Design review of the part built by this model. Coordinates are the model's own, in mm. Face numbers are marked on the shaded views. A direction names the side the tool comes from. Coordinates: 2 decimals unless noted, no trailing zeros. Order: outer loops, then holes, each group sorted by start corner. A loop starts at its lowest first (then second) coordinate and runs counter-clockwise, first axis right, second up. Notation, with made-up numbers: (-39.75, 12) -> (13.25, 12) arc R22 cw to (13.25, 37) -> close; hole circle Ø11 at (48, 61). An arc over 180 degrees is marked (long way). Use a Markdown table: item, result. Add a question column.
Q1. Wall thickness on probe 1 along Y at (x, z) = (-29, -15); probe 2 along Y at (x, z) = (5.5, -2.5); probe 3 along X at (y, z) = (20, -0.5): over which ranges is each line inside the solid? List them lowest first.
Q2. Add section D-D (y = 48.5). State the section outline as (x, z) points.
Q3. Add section C-C (y = -14). State the section outline as (x, z) points, then the cut area to 3 significant figures.
Q4. The part is to be moulded in two halves that separate along X. For the marked faces 1, 2, 3 and 4, say which applies: pulls with the +X half, pulls with the -X half, needs draft (parallel to the pull), parting line crosses it, or undercut.
Q5. Insertion check: pin 1 (6 mm diameter, centred on x = -4.5, y = 3.5, fed in from +Z); pin 2 (8.5 mm diameter, centred on x = -21, y = -3, fed in from +Z); pin 3 (2 mm diameter, centred on x = -37, z = -35, fed in from +Y) (3 decimals); pin 4 (1.5 mm diameter, centred on x = -10.5, y = -11.5, fed in from +Z). Each pin has a flat end and moves straight along its axis. Give the tip position at first contact, or say it passes through.
Q6. Machinability: for the marked faces 5, 6, 7, 8 and 9, which of the approach directions +Z, -Z, +X, -X, +Y, -Y give a long, thin tool a straight path to every point of the face, cutting with its end or side? Answer none if there is none.
Autodesk Inventor part; units mm, degrees
ref_plane "YZ Plane" through (0, 0, 0) normal (1, 0, 0) x (0, 1, 0)
ref_plane "XZ Plane" through (0, 0, 0) normal (0, 1, 0) x (-1, 0, 0)
ref_plane "XY Plane" through (0, 0, 0) normal (0, 0, 1) x (1, 0, 0)
sketch "Sketch1" plane through (0, 0, 0) normal (0, 0, 1) x (1, 0, 0)
  line L0 (0, 0) -> (0, 60.96)
  line L1 (0, 60.96) -> (25.4, 60.96)
  arc A0 (28.575, 57.785) -> (25.4, 60.96) centre (25.4, 57.785) ccw
  line L2 (28.575, 57.785) -> (28.575, 0)
  line L3 (28.575, 0) -> (0, 0)
  dimension "d0" = 3.175
  dimension "d1" = 60.96
  dimension "d3" = 28.575
revolve "Can" add sketch "Sketch1" angle 360 about axis through (0, 0, 0) along (0, 1, 0)
sketch "Sketch2" plane through (0, 0, 0) normal (0, -1, 0) x (1, 0, 0)
  circle A0 centre (0, 0) radius 28.575
  circle A1 centre (0, 0) radius 34.036
  line L0 (-26.3398, 32.6898) -> (26.3398, 32.6898)
  line L1 (32.6898, 26.3398) -> (32.6898, -26.3398)
  line L2 (26.3398, -32.6898) -> (-26.3398, -32.6898)
  line L3 (-32.6898, -26.3398) -> (-32.6898, 26.3398)
  arc A2 (32.6898, 26.3398) -> (26.3398, 32.6898) centre (26.3398, 26.3398) ccw
  arc A3 (-26.3398, 32.6898) -> (-32.6898, 26.3398) centre (-26.3398, 26.3398) ccw
  arc A4 (-32.6898, -26.3398) -> (-26.3398, -32.6898) centre (-26.3398, -26.3398) ccw
  arc A5 (26.3398, -32.6898) -> (32.6898, -26.3398) centre (26.3398, -26.3398) ccw
  point P0 (-32.6898, 32.6898)
  point P1 (32.6898, 32.6898)
  point P2 (0, 32.6898)
  point P3 (-32.6898, 0)
  dimension "d5" = 65.3796
  dimension "d6" = 68.072
  dimension "d7" = 6.35
extrude "Plate" add sketch "Sketch2" along normal blind 10.3632 contours A0 | A1 L1 | L1 A1 L2 L3 L0 | A1 L0 A2 L1 | L1 A5 L2 A1 | L0 A1 | A1 L2 | A1 L3 A3 L0 | L2 A4 L3 A1 | L3 A1
sketch "Sketch3" plane through (0, -10.3632, 0) normal (0, -1, 0) x (1, 0, 0)
  arc A0 (-9.4777, -32.6898) -> (9.4777, -32.6898) centre (0, 0) ccw
  circle A1 centre (-16.1798, 0) radius 2.413
  circle A2 centre (16.1798, 0) radius 2.413
  dimension "d10" = 4.826
  dimension "d11" = 32.3596
  dimension "d12" = 16.1798
extrude "Coil Studs" add sketch "Sketch3" along normal blind 9.525
thread "Coil Stud 1"
thread "Coil Stud 2"
sketch "Sketch4" plane through (0, -10.3632, 0) normal (0, -1, 0) x (1, 0, 0)
  arc A0 (-9.4777, -32.6898) -> (9.4777, -32.6898) centre (0, 0) ccw
  circle A1 centre (0, 14.6812) radius 3.9688
  circle A2 centre (0, -14.6812) radius 3.9688
  dimension "d19" = 29.3624
  dimension "d20" = 14.6812
  dimension "d21" = 7.9375
extrude "Power Studs" add sketch "Sketch4" along normal blind 15.0876
thread "Power Stud 1"
thread "Power Stud 2"
ref_plane "Work Plane1" through (0, 15.24, 0) normal (0, 1, 0) x (1, 0, 0)
sketch "Sketch5" plane through (0, 15.24, 0) normal (0, 1, 0) x (1, 0, 0)
  line L0 (-37.592, 12.4714) -> (-19.05, 12.4714)
  line L1 (-19.05, 12.4714) -> (-19.05, -12.4714)
  line L2 (-19.05, -12.4714) -> (-37.592, -12.4714)
  line L3 (-37.592, -12.4714) -> (-37.592, 12.4714)
  point P0 (0, 0)
  point P1 (-19.05, 0)
  dimension "d29" = 37.592
  dimension "d30" = 24.9428
  dimension "d31" = 19.05
extrude "Extrusion4" add sketch "Sketch5" along normal blind 34.925
sketch "Sketch6" plane through (0, 50.165, 0) normal (0, 1, 0) x (1, 0, 0)
  arc A0 (-25.7098, 12.4714) -> (-25.7098, -12.4714) centre (0, 0) ccw
  line L0 (-37.592, 12.4714) -> (-25.7098, 12.4714)
  line L1 (-25.7098, -12.4714) -> (-37.592, -12.4714)
  line L2 (-37.592, 12.4714) -> (-35.7632, 12.4714)
  line L3 (-35.7632, 13.97) -> (-35.7632, 39.6951)
  line L4 (-35.7632, 39.6951) -> (-37.592, 39.6951)
  line L5 (-37.592, 39.6951) -> (-37.592, 12.4714)
  circle A1 centre (0, 0) radius 28.575
  arc A2 (-26.8755, -13.97) -> (-26.8755, 13.97) centre (0, 0) ccw
  line L6 (-35.7632, 13.97) -> (-26.8755, 13.97)
  line L7 (-37.592, -12.4714) -> (-35.7632, -12.4714)
  line L8 (-35.7632, -13.97) -> (-35.7632, -39.6951)
  line L9 (-35.7632, -39.6951) -> (-37.592, -39.6951)
  line L10 (-37.592, -39.6951) -> (-37.592, -12.4714)
  line L11 (-35.7632, -13.97) -> (-26.8755, -13.97)
  dimension "d34" = 57.15
  dimension "d35" = 60.579
  dimension "d36" = 27.94
  dimension "d37" = 1.8288
  dimension "d38" = 79.3902
extrude "Mounting Plate" add sketch "Sketch6" against normal blind 34.925 contours L0 L5 L4 L3 L6 A2 L11 L8 L9 L10 L1 A1
sketch "Sketch7" plane through (-37.592, 15.24, -39.6951) normal (-1, 0, 0) x (0, 0, 1)
  line L0 (0, 34.925) -> (79.3902, 34.925)
  line L1 (0, 34.925) -> (0, 0)
  line L2 (0, 0) -> (79.3902, 0)
  line L3 (79.3902, 34.925) -> (79.3902, 0)
  circle A0 centre (12.7, 17.4625) radius 3.5687
  line L4 (0, 21.0312) -> (12.7, 21.0312)
  line L5 (12.7, 21.0312) -> (12.7, 13.8938)
  line L6 (12.7, 13.8938) -> (0, 13.8938)
  line L7 (0, 13.8938) -> (0, 21.0312)
  line L8 (0, 31.75) -> (3.175, 34.925)
  line L9 (0, 17.4625) -> (79.3902, 17.4625)
  line L10 (39.6951, 34.925) -> (39.6951, 0)
  circle A1 centre (66.6902, 17.4625) radius 3.5687
  line L11 (79.3902, 21.0312) -> (66.6902, 21.0312)
  line L12 (66.6902, 21.0312) -> (66.6902, 13.8938)
  line L13 (66.6902, 13.8938) -> (79.3902, 13.8938)
  line L14 (79.3902, 13.8938) -> (79.3902, 21.0312)
  line L15 (0, 3.175) -> (3.175, 0)
  line L16 (79.3902, 3.175) -> (76.2152, 0)
  line L17 (76.2152, 34.925) -> (79.3902, 31.75)
  point P0 (39.6951, -15.24)
  dimension "d41" = 7.1374
  dimension "d42" = 12.7
  dimension "d43" = 3.175
  dimension "d44" = 3.175
extrude "Extrusion6" cut sketch "Sketch7" against normal up to next contours L0 L8 L1 | L4 A0 L9 L1 | L0 L3 L17 | L9 A0 L6 L1 | L5 L9 A0 | A0 L9 L5 | A0 L5 L9 | A1 L12 L9 | L9 L12 A1 | L9 L5 A0 | L3 L9 A1 L11 | L12 A1 L9 | L9 A1 L12 | A1 L9 L3 L13 | L2 L1 L15 | L16 L3 L2
equation "\"d12\" = 0.5 * d11"
equation "\"d20\" = 0.5 * d19"
properties part number "realy"
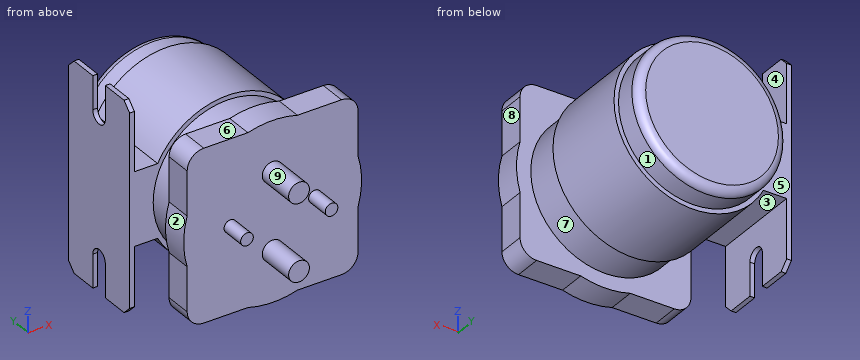
Established:
| question | item | result |
|---|---|---|
| 1 | probe 1 | -10.36 to 0 |
| 1 | probe 2 | -10.36 to 60.96 |
| 1 | probe 3 | -37.59 to 30.29 |
| 2 | outline | (-37.59, -38.19) -> (-35.76, -38.19) -> (-35.76, -13.97) -> (-26.88, -13.97) arc R30.29 ccw (long way) to (-26.88, 13.97) -> (-35.76, 13.97) -> (-35.76, 38.19) -> (-37.59, 38.19) -> close |
| 3 | outline | circle Ø4.83 at (-16.18, 0); circle Ø7.94 at (0, -14.68); circle Ø7.94 at (0, 14.68); circle Ø4.83 at (16.18, 0) |
| 3 | area | 136 mm^2 |
| 4 | face 1 | parting line crosses it |
| 4 | face 2 | pulls with the -X half |
| 4 | face 3 | undercut |
| 4 | face 4 | undercut |
| 5 | pin 1 | z = 28.54 |
| 5 | pin 2 | z = 32.69 |
| 5 | pin 3 | y = 50.165 |
| 5 | pin 4 | through |
| 6 | face 5 | +Y |
| 6 | face 6 | +Z, -X, +Y, -Y |
| 6 | face 7 | none |
| 6 | face 8 | +Z, +X, +Y, -Y |
| 6 | face 9 | -Y |
